from build123d import *

# Parameters (mm, degrees)
SKETCH1_W                  = 130.5
SKETCH1_H                  = 10
SKETCH1_W_2                = 10
SKETCH1_H_2                = 85.5
BOSS_EXTRUDE1_DEPTH        = 3
M2_5_CLEARANCE_HOLE1_D     = 2.9
M2_5_CLEARANCE_HOLE1_DEPTH = 3
M2_5_CLEARANCE_HOLE1_TIP   = 0.871247898
M2_5_CLEARANCE_HOLE2_D     = 2.9
M2_5_CLEARANCE_HOLE2_DEPTH = 3
M2_5_CLEARANCE_HOLE2_TIP   = 0.871247898
M2_5_CLEARANCE_HOLE3_D     = 2.9
M2_5_CLEARANCE_HOLE3_DEPTH = 3
M2_5_CLEARANCE_HOLE3_TIP   = 0.871247898
M2_5_CLEARANCE_HOLE4_D     = 2.9
M2_5_CLEARANCE_HOLE4_DEPTH = 3
M2_5_CLEARANCE_HOLE4_TIP   = 0.871247898


with BuildPart() as part:
    # Sketch1 → Boss-Extrude1 (new body)
    with BuildSketch(Plane(origin=(0, 0, 0), x_dir=(1, 0, 0), z_dir=(0, 1, 0))):
        with Locations((40.207417437, 2.647058824)):
            Rectangle(SKETCH1_W, SKETCH1_H)
        with Locations((40.207417437, 2.647058824)):
            Rectangle(SKETCH1_W_2, SKETCH1_H_2)
    extrude(amount=BOSS_EXTRUDE1_DEPTH)

    # M2.5 Clearance Hole1
    with Locations(Plane(origin=(0, 3, 0), x_dir=(1, 0, 0), z_dir=(0, 1, 0))):
        with Locations((-23.042582563, 2.647058824)):
            Hole(M2_5_CLEARANCE_HOLE1_D / 2, depth=M2_5_CLEARANCE_HOLE1_DEPTH)
            with Locations((0, 0, -(M2_5_CLEARANCE_HOLE1_DEPTH + M2_5_CLEARANCE_HOLE1_TIP / 2))):  # 118° drill point
                Cone(0, M2_5_CLEARANCE_HOLE1_D / 2, M2_5_CLEARANCE_HOLE1_TIP, mode=Mode.SUBTRACT)

    # M2.5 Clearance Hole2
    with Locations(Plane(origin=(0, 3, 0), x_dir=(1, 0, 0), z_dir=(0, 1, 0))):
        with Locations((40.207417437, 43.397058824)):
            Hole(M2_5_CLEARANCE_HOLE2_D / 2, depth=M2_5_CLEARANCE_HOLE2_DEPTH)
            with Locations((0, 0, -(M2_5_CLEARANCE_HOLE2_DEPTH + M2_5_CLEARANCE_HOLE2_TIP / 2))):  # 118° drill point
                Cone(0, M2_5_CLEARANCE_HOLE2_D / 2, M2_5_CLEARANCE_HOLE2_TIP, mode=Mode.SUBTRACT)

    # M2.5 Clearance Hole3
    with Locations(Plane(origin=(0, 3, 0), x_dir=(1, 0, 0), z_dir=(0, 1, 0))):
        with Locations((103.457417437, 2.647058824)):
            Hole(M2_5_CLEARANCE_HOLE3_D / 2, depth=M2_5_CLEARANCE_HOLE3_DEPTH)
            with Locations((0, 0, -(M2_5_CLEARANCE_HOLE3_DEPTH + M2_5_CLEARANCE_HOLE3_TIP / 2))):  # 118° drill point
                Cone(0, M2_5_CLEARANCE_HOLE3_D / 2, M2_5_CLEARANCE_HOLE3_TIP, mode=Mode.SUBTRACT)

    # M2.5 Clearance Hole4
    with Locations(Plane(origin=(0, 3, 0), x_dir=(1, 0, 0), z_dir=(0, 1, 0))):
        with Locations((40.207417437, -38.102941176)):
            Hole(M2_5_CLEARANCE_HOLE4_D / 2, depth=M2_5_CLEARANCE_HOLE4_DEPTH)
            with Locations((0, 0, -(M2_5_CLEARANCE_HOLE4_DEPTH + M2_5_CLEARANCE_HOLE4_TIP / 2))):  # 118° drill point
                Cone(0, M2_5_CLEARANCE_HOLE4_D / 2, M2_5_CLEARANCE_HOLE4_TIP, mode=Mode.SUBTRACT)


solid = part.part
Can you work these out from the model? Positions are in its coordinate system, mm. A direction names the side the tool comes from. Round coordinates to 2 decimals unless told otherwise and drop trailing zeros. Write each loop counter-clockwise with the first axis right and the second up, starting at its lowest first coordinate (ties: lowest second). Pieces come first, ordered by that corner, then holes. Notation, with made-up numbers: (-18, 20) -> (2, 20) arc R29 ccw to (2, 51) -> close; hole circle Ø1 at (32, -0.75). An arc over 180 degrees is marked (long way). One line per question, with ' | ' between items. Start each with the question number.
1) Suppose I cut it at B-B on z = -24.5. Write out the boundary of the cut face in (x, y).
2) Suppose I cut it at C-C on x = 14.5. Write out the boundary of the cut face in (y, z), then the cut area to 3 significant figures.
3) Suppose I cut it at A-A on y = 2.55. Write out the boundary of the cut face in (x, z), then the cut area to 3 significant figures.
4) I need wall thicknesses on line 1 (Z direction, x = 94.5, y = 1.25); line 2 (X direction, y = 1.9, z = 25.5). Which ranges of each line are inside material? Lowest first, please. Write a range as [from, to].
5) If we mould it in two halves opening along X, with no side actions, what happens to faces 4 (the cylindrical face through (40.52, 1.48, 39.52)), 5 (the flat face through (35.207, 1, 21)), 6 (the flat face through (5, 1, -7.647))? For each: released by +X, released by -X, zero draft, split by the parting line, or undercut.
6) I'm going to push flat-ended pins straight in: P1, Ø0.9, axis at x = 17, y = 1, coming from the -Z side; P2, Ø1.5, axis at y = 2.5, z = 15, coming from the -X side; P3, Ø0.9, axis at y = 2, z = -20.5, coming from the +X side. Where does each tip first touch, or does it pass through?
7) On a 3-axis mill with a long thin cutter (end or side, diameter ignored), from which of +Z, -Z, +X, -X, +Y, -Y can I reach the whole of each face in a straight line? I mean faces 1 (the flat face through (75, 1, 2.353)), 2 (the flat face through (5, 1, 2.353)), 3 (the flat face through (75, 1, -7.647)). Say none if no direction works.
Return value:
1) outline: (35.21, 0) -> (45.21, 0) -> (45.21, 3) -> (35.21, 3) -> close
2) outline: (0, -7.65) -> (3, -7.65) -> (3, 2.35) -> (0, 2.35) -> close | area: 30.0 mm2
3) outline: (-25.04, -7.65) -> (35.21, -7.65) -> (35.21, -45.4) -> (45.21, -45.4) -> (45.21, -7.65) -> (105.46, -7.65) -> (105.46, 2.35) -> (45.21, 2.35) -> (45.21, 40.1) -> (35.21, 40.1) -> (35.21, 2.35) -> (-25.04, 2.35) -> close; hole circle Ø2.9 at (-23.04, -2.65); hole circle Ø2.9 at (40.21, -43.4); hole circle Ø2.9 at (40.21, 38.1); hole circle Ø2.9 at (103.46, -2.65) | area: 2,030 mm2
4) line 1: z = [-7.65, 2.35] | line 2: x = [35.21, 45.21]
5) face 4: undercut | face 5: released by -X | face 6: zero draft
6) P1: stops at z = -7.65 | P2: stops at x = 35.21 | P3: stops at x = 45.21
7) face 1: +Z, +X, +Y, -Y | face 2: +Z, -X, +Y, -Y | face 3: -Z, +X, +Y, -Y
